The model under review builds one solid part; all positions refer to its coordinate system, in mm. Face numbers are marked on the shaded views. Round coordinates to 2 decimals unless told otherwise and drop trailing zeros. Order: outer loops, then holes, each group sorted by start corner. A loop starts at its lowest first (then second) coordinate and runs counter-clockwise, first axis right, second up. Notation, with made-up numbers: M 75.5,69.25 L 100.5,69.25 A30 ccw 100.5,99.25 Z; hole C 37.25,-17.5 d2. An arc over 180 degrees is marked long. Use a Markdown table: item, result. Add a question column.
1. Consider section B-B on z = 21.5. State the section outline as (x, y) points.
2. The part is to be moulded in two halves that separate along Y. For the marked faces 1, 2, 3 and 4, say which applies: +Y half, -Y half, draft (parallel to the pull), parting line (faces both ways), or undercut.
3. To check wall thickness, follow probe 1 along Y at (x, z) = (-53.5, 24.5); probe 2 along X at (y, z) = (-53, 4); probe 3 along X at (y, z) = (-81, 25). State the ranges of each line that lie inside material, in increasing order.
4. Insertion check: P1, Ø0.8, axis at y = -96.5, z = 27.5, coming from the -X side; P2, Ø1.5, axis at x = -66.5, z = 5, coming from the +Y side; P3, Ø1, axis at y = -74, z = 24.5, coming from the +X side. Each pin has a flat end and moves straight along its axis. Give the tip position at first contact, or say it passes through.
5. Consider section D-D on x = -72. Count the separate pieces of the cut face and the enclosed holes in it, then the cut area to 3 significant figures.
6. Consider section A-A on y = -73.5. State the section outline as (x, z) points, then the cut area to 3 significant figures.
7. Consider section C-C on y = -82. State the section outline as (x, z) points.
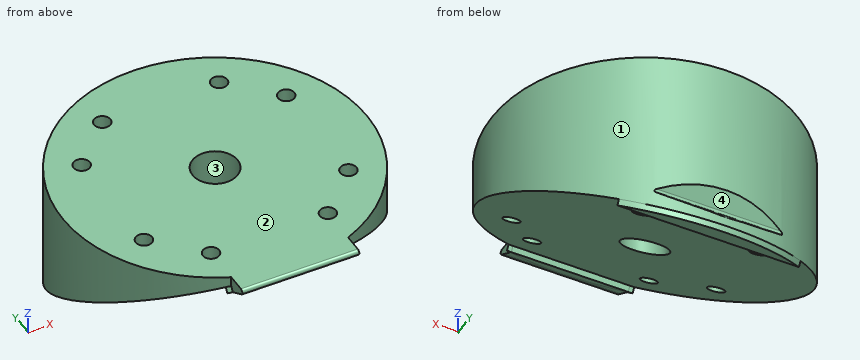
Autodesk Inventor part; units mm, degrees
ref_plane "Arbeitsebene5" through (-88.1514, -83.8908, 20.4259) normal (0, 0.5, 0.8660254) x (1, 0, 0)
ref_plane "YZ Plane" through (0, 0, 0) normal (1, 0, 0) x (0, 1, 0)
ref_plane "XZ Plane" through (0, 0, 0) normal (0, 1, 0) x (-1, 0, 0)
ref_plane "Work Plane1" through (-54.6514, -58.9369, 28.8009) normal (0, 0, -1) x (-1, 0, 0)
ref_plane "Arbeitsebene5" through (-88.1514, -83.8908, 20.4259) normal (0, 0.5, 0.8660254) x (1, 0, 0)
sketch "Sketch1" plane through (-50.6514, -58.9369, 28.8009) normal (0, 0, 1) x (1, 0, 0)
  circle A0 centre (-11.9999, -12.4979) radius 25.9979
  circle A1 centre (-2, 4.9999) radius 1.3999
  circle A2 centre (-22, 5) radius 1.4
  circle A3 centre (-12, -12.5) radius 3.85
  line L0 (-5, -5) -> (-5, 0)
  line L1 (0, 0) -> (0, -5)
  circle A4 centre (-22, -30) radius 1.4
  circle A5 centre (-2, -30) radius 1.4001
  line L2 (-5, 0) -> (0, 0)
  line L3 (0, 0) -> (0, -5)
  line L4 (0, -5) -> (-5, -5)
  line L5 (-5, -5) -> (-5, 0)
  circle A6 centre (-12, -12.5) radius 4
  point P0 (50.6514, 58.9369)
  dimension "d2" = 8
extrude "Extrusion1" add sketch "Sketch1" against normal up to surface contours A0 | L0 L2 L1 L4 | A6 surface through (-88.1514, -83.8908, 20.4259) normal (0, 0.5, 0.8660254)
sketch "Skizze17" plane through (-62.6512, -71.4348, 13.2343) normal (0, -0.5, -0.8660254) x (-1, 0, 0)
  line L0 (23.5002, 23.867) -> (-23.4998, 23.867)
  arc A0 (-23.4998, 23.867) -> (-25.4998, 21.867) centre (-23.4998, 21.867) ccw
  line L1 (-25.4998, 21.867) -> (-25.4998, -25.133)
  arc A1 (-25.4998, -25.133) -> (-23.4998, -27.133) centre (-23.4998, -25.133) ccw
  line L2 (-23.4998, -27.133) -> (23.5002, -27.133)
  arc A2 (23.5002, -27.133) -> (25.5002, -25.133) centre (23.5002, -25.133) ccw
  line L3 (25.5002, -25.133) -> (25.5002, 21.867)
  arc A3 (25.5002, 21.867) -> (23.5002, 23.867) centre (23.5002, 21.867) ccw
  line L4 (-17.4998, 11.367) -> (17.5002, 11.367)
  line L5 (17.5002, 11.367) -> (17.5002, -12.633)
  line L6 (17.5002, -12.633) -> (-17.4998, -12.633)
  line L7 (-17.4998, -12.633) -> (-17.4998, 11.367)
  line L8 (-23.4998, 24.067) -> (23.5002, 24.067)
  arc A4 (25.7002, 21.867) -> (23.5002, 24.067) centre (23.5002, 21.867) ccw
  line L9 (25.7002, 21.867) -> (25.7002, -25.133)
  arc A5 (23.5002, -27.333) -> (25.7002, -25.133) centre (23.5002, -25.133) ccw
  line L10 (23.5002, -27.333) -> (-23.4998, -27.333)
  arc A6 (-25.6998, -25.133) -> (-23.4998, -27.333) centre (-23.4998, -25.133) ccw
  line L11 (-25.6998, -25.133) -> (-25.6998, 21.867)
  arc A7 (-23.4998, 24.067) -> (-25.6998, 21.867) centre (-23.4998, 21.867) ccw
  ellipse E0 centre (-9.9998, 20.2048) end of major axis (-9.9998, 21.8213) minor radius 1.3999
  ellipse E1 centre (10.0001, 20.2048) end of major axis (10.0001, 21.8213) minor radius 1.4
  ellipse E2 centre (0.0001, -0.0025) end of major axis (0.0001, 4.4432) minor radius 3.85
  ellipse E3 centre (10.0001, -20.2097) end of major axis (10.0001, -18.5931) minor radius 1.4
  ellipse E4 centre (-9.9999, -20.2096) end of major axis (-9.9999, -18.593) minor radius 1.4001
  ellipse E5 centre (0, 0) end of major axis (0, -30.0198) minor radius 25.9979
  point P0 (-62.6512, 68.4815)
  point P1 (15.5395, 24.067)
  point P2 (-15.5395, 24.067)
  point P3 (10.7503, -27.333)
  point P4 (-10.7503, -27.333)
  dimension "d65" = 0.2
extrude "Extrusion13" add sketch "Skizze17" along normal blind 1 contours L8 E5 | E5 L10
ref_plane "Arbeitsebene6" through (-62.6514, -59.1868, 48.3009) normal (-1, 0, 0) x (0, 0, -1)
sketch "Skizze18" plane through (-62.6514, -59.1868, 48.3009) normal (-1, 0, 0) x (0, 0, -1)
  line L0 (47.1, -8.5947) -> (47.1, -8.5947)
  line L1 (47.1, -8.5947) -> (47.966, -8.0947)
  line L2 (47.966, -8.0947) -> (47.966, -8.0947)
  line L3 (47.1, -8.5947) -> (47.966, -8.0947)
  line L4 (21.4, 35.919) -> (21.4, 35.919)
  line L5 (21.4, 35.919) -> (22.266, 36.419)
  line L6 (22.266, 36.419) -> (22.266, 36.419)
  line L7 (21.4, 35.919) -> (22.266, 36.419)
  line L8 (21.4, 35.919) -> (22.266, 36.419)
  line L9 (22.266, 36.419) -> (19.5, 34.8221)
  line L10 (19.5, 38.2458) -> (19.5, -13.75)
  line L11 (22.266, 36.419) -> (19.5, 34.8221)
  line L12 (22.266, 36.419) -> (20.9226, 38.7458)
  line L13 (22.266, 36.419) -> (20.433, 39.5939)
  line L14 (19.5, 39.3439) -> (19.5, 34.8221)
  arc A0 (20.433, 39.5939) -> (19.5, 39.3439) centre (20, 39.3439) ccw
  point P0 (48.3009, -59.1868)
  point P1 (19.5, 38.2458)
  point P2 (20.9226, 38.7458)
  dimension "d68" = 0.5
extrude "Extrusion14" add sketch "Skizze18" along normal mid plane 20
sketch "Skizze19" plane through (-62.6514, -59.1868, 48.3009) normal (-1, 0, 0) x (0, 0, -1)
  line L0 (47.1, -8.5947) -> (47.1, -8.5947)
  line L1 (47.1, -8.5947) -> (47.966, -8.0947)
  line L2 (47.966, -8.0947) -> (47.966, -8.0947)
  line L3 (47.1, -8.5947) -> (47.966, -8.0947)
  line L4 (48.1255, -13.6035) -> (46.0052, -11.4832)
  line L5 (48.4791, -13.75) -> (51.4776, -13.75) construction
  line L6 (45.2981, -11.4832) -> (43.0314, -13.75)
  line L7 (19.5, -13.75) -> (50.0764, -13.75)
  line L8 (43.0314, -13.75) -> (48.272, -13.75)
  arc A0 (46.0052, -11.4832) -> (45.2981, -11.4832) centre (45.6517, -11.8368) ccw
  arc A1 (48.1255, -13.6035) -> (48.4791, -13.75) centre (48.4791, -13.25) ccw
  point P0 (48.3009, -59.1868)
  point P1 (48.4791, -13.75)
  dimension "d71" = 135
  dimension "d72" = 90
  dimension "d73" = 0.5
extrude "Extrusion15" cut sketch "Skizze19" along normal through all both and the other way through all
sketch "Skizze20" plane through (-50.6514, -58.9369, 28.8009) normal (0, 0, 1) x (1, 0, 0)
  circle A0 centre (-29.4977, -2.4981) radius 1.3999
  circle A1 centre (-29.4977, -22.498) radius 1.4
  circle A2 centre (-11.9977, -12.498) radius 3.85
  circle A3 centre (5.5022, -22.498) radius 1.4
  circle A4 centre (5.5022, -2.498) radius 1.4001
  arc A5 (-2.0001, -36.4957) -> (-22.0001, -36.4955) centre (-11.9999, -12.4979) ccw
  line L0 (-22.0001, -39.5939) -> (-22.0001, -36.4955)
  line L1 (-22.0001, -39.5939) -> (-2.0001, -39.5939)
  line L2 (-2.0001, -36.4957) -> (-2.0001, -39.5939)
  line L3 (5.498, -22.4977) -> (5.498, -2.4981)
  line L4 (5.498, -2.4981) -> (-29.4977, -2.4981)
  line L5 (-29.4977, -2.4981) -> (-29.4977, -22.4977)
  line L6 (-29.4977, -22.4977) -> (5.498, -22.4977)
  line L7 (5.498, -22.4977) -> (-29.4977, -2.4981) construction
  line L8 (5.498, -2.4981) -> (-29.4977, -22.4977) construction
  point P0 (50.6514, 58.9369)
hole "Bohrung3" at (-80.1491, -61.4349, 28.8009) at (-80.1491, -81.4346, 28.8009) at (-45.1491, -81.4349, 28.8009) at (-45.1534, -61.4349, 28.8009) direction (0, 0, -1) diameter 2.8 depth 14 tip angle 118
properties part number "Spectrometer_gratingholder_v0"
Answer block:
| question | item | result |
|---|---|---|
| 1 | outline | M -84.35,-85.75 L -40.95,-85.75 A26 ccw long Z; hole C -80.15,-81.43 d2.8; hole C -80.15,-61.43 d2.8; hole C -72.65,-53.94 d2.8; hole C -62.65,-71.44 d7.7; hole C -52.65,-53.94 d2.8; hole C -45.15,-81.43 d2.8; hole C -45.15,-61.43 d2.8 |
| 2 | face 1 | parting line |
| 2 | face 2 | draft |
| 2 | face 3 | undercut |
| 2 | face 4 | +Y half |
| 3 | probe 1 | -90.95 to -90.05, -87.82 to -55.05, -52.82 to -47.1 |
| 3 | probe 2 | -80.98 to -73.69, -71.61 to -53.69, -51.61 to -44.32 |
| 3 | probe 3 | -86.83 to -81.48, -78.82 to -46.48, -43.82 to -38.48 |
| 4 | P1 | x = -72.65 |
| 4 | P2 | y = -45.62 |
| 4 | P3 | x = -36.74 |
| 5 | separate pieces | 3 |
| 5 | enclosed holes | 0 |
| 5 | area | 687 mm^2 |
| 6 | outline | M -88.57,14.43 L -65.9,14.43 L -65.9,28.8 L -88.57,28.8 Z; M -59.4,14.43 L -36.74,14.43 L -36.74,28.8 L -59.4,28.8 Z |
| 6 | area | 652 mm^2 |
| 7 | outline | M -86.41,19.33 L -81.43,19.33 L -81.43,28.8 L -86.41,28.8 Z; M -78.87,19.33 L -46.43,19.33 L -46.43,28.8 L -78.87,28.8 Z; M -43.87,19.33 L -38.9,19.33 L -38.9,28.8 L -43.87,28.8 Z |
